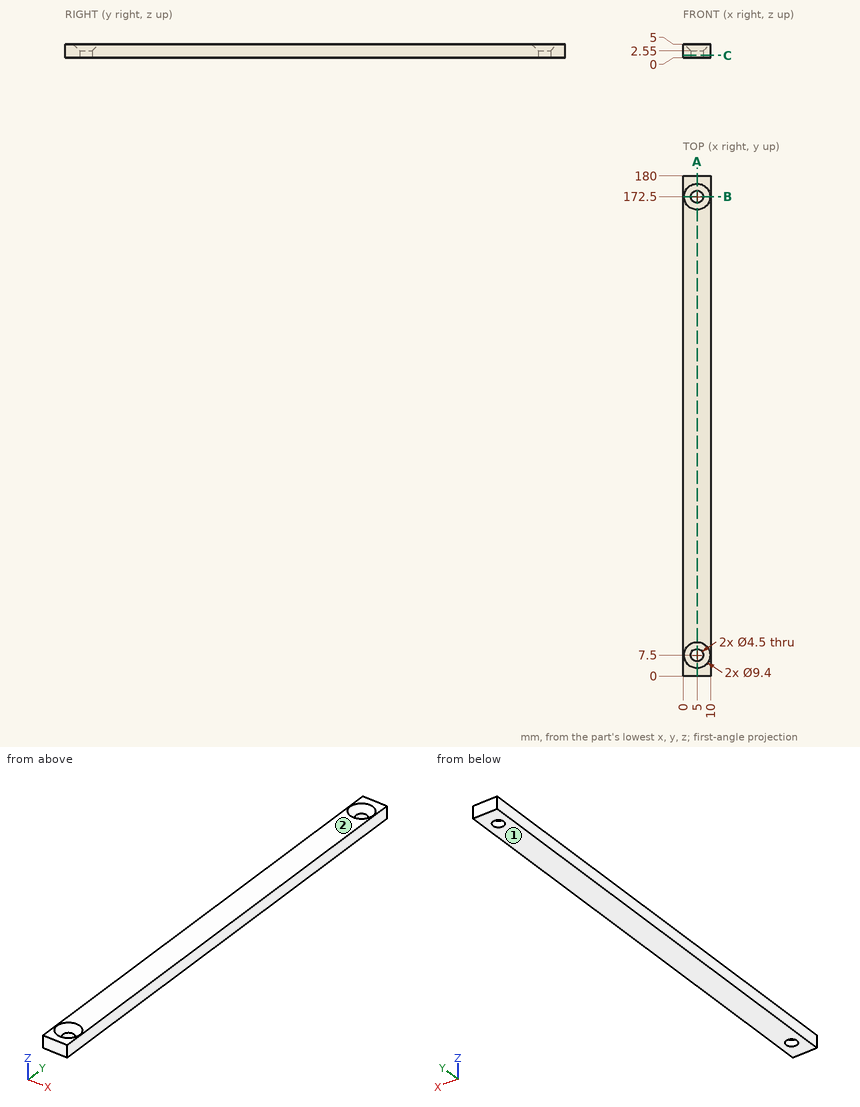
Here's the drawing with two shaded views (mm, measured from the low corner). I have some questions. Coordinates: 2 decimals unless noted, no trailing zeros. Order: outer loops, then holes, each group sorted by start corner. A loop starts at its lowest first (then second) coordinate and runs counter-clockwise, first axis right, second up. Notation, with made-up numbers: M 25.25,-10.5 L 30.25,-10.5 A33 cw 30.25,24.5 Z; hole C 3.5,29 d5. An arc over 180 degrees is marked long. Write item = value, one per line.
(1) For pin 1 Ø2 at (y, z) = (123.5, 2) entering from -X, with a flat end and sliding along its axis, tell me the tip position at first contact or that it passes through.
Results are:
pin_1 = 0
(2) Suppose I cut it at B-B on y = 172.5. Please give me the cut outline in (x, z), plus the area to 3 significant figures.
Results are:
outline = M 0,0 L 2.75,0 L 2.75,2.55 L 0.3,5 L 0,5 Z; M 7.25,0 L 10,0 L 10,5 L 9.7,5 L 7.25,2.55 Z
area = 21.5 mm2
(3) If we mould it in two halves opening along Z, with no side actions, what happens to the marked faces 1 and 2? For each: pulls with the +Z half, pulls with the -Z half, needs draft (parallel to the pull), parting line crosses it, or undercut.
Results are:
face_1 = pulls with the -Z half
face_2 = pulls with the +Z half
(4) Suppose I cut it at C-C on z = 0.9. Please give me the cut outline in (x, y), plus the area to 3 significant figures.
Results are:
outline = M 0,0 L 10,0 L 10,180 L 0,180 Z; hole C 5,7.5 d4.5; hole C 5,172.5 d4.5
area = 1,770 mm2
(5) Suppose I cut it at A-A on x = 5. Please give me the cut outline in (y, z), plus the area to 3 significant figures.
Results are:
outline = M 0,0 L 5.25,0 L 5.25,2.55 L 2.8,5 L 0,5 Z; M 9.75,0 L 170.25,0 L 170.25,2.55 L 167.8,5 L 12.2,5 L 9.75,2.55 Z; M 174.75,0 L 180,0 L 180,5 L 177.2,5 L 174.75,2.55 Z
area = 843 mm2
(6) I need wall thicknesses on line 1 along Y through (x, z) = (5, 2); line 2 along X through (y, z) = (172.5, 1.75); line 3 along Y through (x, z) = (7, 1.7). Which ranges of each line are inside material? Lowest first, please. Write a range as [from, to].
Results are:
line_1 = [0, 5.25], [9.75, 170.25], [174.75, 180]
line_2 = [0, 2.75], [7.25, 10]
line_3 = [0, 6.47], [8.53, 171.47], [173.53, 180]
